For this review, take the finished solid that the model builds, in its own axes (mm). Coordinates: 2 decimals unless noted, no trailing zeros. Answer as a JSON object with one key per item and string values. Group by question number.
Item 1: Clearance check with a flat-ended pin moving along its axis: pin 1 (1.5 mm diameter, centred on x = 21, y = -3.5, fed in from +Z). State where the tip first meets the part, or that it passes through.
Item 2: Mouldability with a two-part tool opening along Y and no side actions: class faces 1 (the cylindrical face through (25.08, -3.7, 0)), 2 (the cylindrical face through (25.1, -4.7, 0)), 3 (the flat face through (34, 2, 0.25)) as released by +Y, released by -Y, zero draft, split by the parting line, or undercut.
Item 3: To check wall thickness, follow line 1 (Y direction, x = 25, z = -0.2); line 2 (Y direction, x = 64.5, z = -0.15); line 3 (Y direction, x = 93.8, z = -0.1). State the ranges of each line that lie inside material, in increasing order.
Item 4: We need section A-A (z = 0.1). State how many separate pieces and enclosed holes the cut face has, then the cut area to 3 significant figures.
from build123d import *

# Parameters (mm, degrees)
EXTRUDE_1_DEPTH     = 0.25
SKETCH_3_R          = 0.3
SKETCH_3_R_2        = 0.2
CUT_EXTRUDE_1_DEPTH = 0.25
EXTRUDE_2_DEPTH     = 0.25
FILLET_1_R          = 0.5


with BuildPart() as part:
    # 草图2 → 凸台-拉伸1 (new, symmetric)
    with BuildSketch(Plane.XY):
        with BuildLine():
            ThreePointArc((94.3, -5.23), (94.279085645, -5.63954323), (94, -5.94))
            add(Edge.make_bspline(
                [(1.4, -2.38), (47.954561827, 5.976867864), (94, -5.94)],
                knots=[0, 0, 0, 1, 1, 1], degree=2))
            add(Edge.make_bspline(
                [(0, 0), (-4.123736473, -1.859487618), (1.4, -2.38)],
                knots=[0, 0, 0, 1, 1, 1], degree=2))
            add(Edge.make_bspline(
                [(0, 0), (47.273266317, 6.255778848), (94.3, -5.23)],
                knots=[0, 0, 0, 1, 1, 1], degree=2))
        make_face()
    extrude(amount=EXTRUDE_1_DEPTH, both=True)

    # 草图3 → 切除-拉伸1 (cut, symmetric)
    with BuildSketch(Plane.XY):
        with Locations((-1, -1.3)):
            Circle(SKETCH_3_R)
        with Locations((8.6, 0.4)):
            Circle(SKETCH_3_R)
        with Locations((25, 1.6)):
            Circle(SKETCH_3_R)
        with Locations((42.4, 1.5)):
            Circle(SKETCH_3_R)
        with Locations((68, -0.5)):
            Circle(SKETCH_3_R_2)
        with Locations((93.8, -5.5)):
            Circle(SKETCH_3_R_2)
    extrude(amount=CUT_EXTRUDE_1_DEPTH, both=True, mode=Mode.SUBTRACT)

    # 草图4 → 凸台-拉伸2 (add, symmetric)
    with BuildSketch(Plane.XY):
        with BuildLine():
            ThreePointArc((22.854587938, 0.396951856), (25.20918356, -4.692698154), (26.83283005, 0.675022949))
            add(Edge.make_bspline(
                [(22.854587938, 0.396951856), (24.844176287, 0.554595418), (26.83283005, 0.675022949)],
                knots=[0, 0, 0, 1, 1, 1], degree=2))
        make_face()
        with BuildLine():
            Line((24.7, 0.277371993), (24.7, -0.2))
            Line((24.7, -0.2), (25.3, -0.2))
            Line((25.3, -0.2), (25.3, 0.277371993))
            ThreePointArc((25.3, 0.277371993), (25, -3.7), (24.7, 0.277371993))
        make_face(mode=Mode.SUBTRACT)
    extrude(amount=EXTRUDE_2_DEPTH, both=True)

    # 圆角1
    fillet_1_edges = [part.edges().sort_by_distance(p)[0] for p in [
        (26.83283005, 0.675022949, -0.125),
        (22.854587938, 0.396951856, -0.125),
    ]]
    fillet(fillet_1_edges, radius=FILLET_1_R)


solid = part.part
Check sheet entries:
{
 "1": {"pin 1": "passes through"},
 "2": {"face 1": "undercut", "face 2": "undercut", "face 3": "zero draft"},
 "3": {"line 1": "y = -4.7 to -3.7, -0.2 to 1.3, 1.9 to 2.07", "line 2": "y = -0.39 to 0.26", "line 3": "y = -5.89 to -5.7, -5.3 to -5.11"},
 "4": {"separate pieces": "1", "enclosed holes": "7", "area": "125 mm2"}
}
